Here's how the part is built. I have some questions about the finished solid (model axes, mm). A direction names the side the tool comes from. Coordinates: 2 decimals unless noted, no trailing zeros. Write each loop counter-clockwise with the first axis right and the second up, starting at its lowest first coordinate (ties: lowest second). Pieces come first, ordered by that corner, then holes.
```python
from build123d import *

# Parameters (mm, degrees)
F_5_16_CLEARANCE_HOLE1_D         = 8.4328
CIRPATTERN1_COUNT                = 12
F_1_2_0_5_DIAMETER_HOLE1_D       = 12.7
F_1_1_5_DIAMETER_HOLE1_D         = 38.1
F_1_1_5_DIAMETER_HOLE1_DEPTH     = 19.05
CIRPATTERN2_COUNT                = 6
CIRPATTERN3_COUNT                = 2
F_1_8_0_125_DIAMETER_HOLE1_D     = 3.175
F_1_8_0_125_DIAMETER_HOLE1_DEPTH = 6.35
F_1_8_0_125_DIAMETER_HOLE1_TIP   = 0.953866233


with BuildPart() as part:
    # Sketch1 → Revolve1 (revolve)
    with BuildSketch(Plane.XY, mode=Mode.PRIVATE) as revolve1_sk:
        Polygon((-88.9, 0), (-88.9, 41.275), (-50.8, 41.275), (-31.75, 60.325), (-12.7, 60.325), (-12.7, 53.975), (0, 53.975), (0, 34.925), (-31.75, 34.925), (-31.75, 22.225), (-50.8, 22.225), (-50.8, 3.175), (-52.3875, 3.175), (-52.3875, 5.715), (-55.9435, 5.715), (-55.9435, 3.175), (-57.15, 3.175), (-57.15, 0), align=None)
    revolve(revolve1_sk.sketch.rotate(Axis((0, 0, 0), (0, 1, 0)), 270), axis=Axis((0, 0, 0), (0, 1, 0)))

    # 5/16 Clearance Hole1 (through all)
    with Locations(Plane(origin=(0, 41.275, 0), x_dir=(1, 0, 0), z_dir=(0, 1, 0))):
        with Locations((-73.603547963, -19.722011237)):
            f_5_16_clearance_hole1 = Hole(F_5_16_CLEARANCE_HOLE1_D / 2)

    # CirPattern1: 5/16 Clearance Hole1 ×12 about axis
    cirpattern1_axis = Axis((0, 0, 0), (0, 1, 0))
    for i in range(1, CIRPATTERN1_COUNT):
        add(f_5_16_clearance_hole1.rotate(cirpattern1_axis, i * 360 / CIRPATTERN1_COUNT), mode=Mode.SUBTRACT)

    # 1/2 (0.5) Diameter Hole1 (through all)
    with Locations(Plane(origin=(0, 60.325, 0), x_dir=(1, 0, 0), z_dir=(0, 1, 0))):
        with Locations((0, 0)):
            Hole(F_1_2_0_5_DIAMETER_HOLE1_D / 2)

    # Sketch11 → 1/2 NPT Tapped Hole1 (revolve, cut)
    with BuildSketch(Plane(origin=(41.275, 50.8, 0), x_dir=(-0.707106781186546, 0.707106781186549, 0), z_dir=(0, 0, 1))):
        Polygon((0, 0), (0, 127.968649725), (8.9281, 127.968649725), (8.9281, 13.462), (9.479726792, 13.462), (9.8827971, 0), align=None)
    revolve(axis=Axis((45.765128061, 55.290128061, 0), (-0.707106781186549, -0.707106781186546, 0)), mode=Mode.SUBTRACT)

    # 1 (1.5) Diameter Hole1
    with Locations(Plane(origin=(0, 60.325, 0), x_dir=(1, 0, 0), z_dir=(0, 1, 0))):
        with Locations((-23.8125, -41.244459855)):
            f_1_1_5_diameter_hole1 = Hole(F_1_1_5_DIAMETER_HOLE1_D / 2, depth=F_1_1_5_DIAMETER_HOLE1_DEPTH)

    # Sketch19 → 3/8 NPT Tapped Hole1 (revolve, cut)
    with BuildSketch(Plane(origin=(-23.8125, 41.275, 41.244459855), x_dir=(0, 0, 1), z_dir=(1, 0, 0))):
        Polygon((0, 0), (0, 26.640582582), (7.1374, 22.352), (7.1374, 10.414), (7.653732494, 10.414), (7.9655416, 0), align=None)
    f_3_8_npt_tapped_hole1 = revolve(axis=Axis((-23.8125, 47.625, 41.244459855), (0, -1, 0)), mode=Mode.SUBTRACT)

    # Sketch21 → Tap Drill for 1/4-20 Tap1 (revolve, cut)
    with BuildSketch(Plane(origin=(21.997045256, 60.325, -12.7), x_dir=(0, 0, 1), z_dir=(1, 0, 0))):
        Polygon((0, 0), (0, 17.535816902), (2.5527, 16.002), (2.5527, 0), align=None)
    tap_drill_for_1_4_20_tap1 = revolve(axis=Axis((21.997045256, 66.675, -12.7), (0, -1, 0)), mode=Mode.SUBTRACT)

    # CirPattern2: Tap Drill for 1/4-20 Tap1 ×6 about axis
    cirpattern2_axis = Axis((0, 0, 0), (0, 1, 0))
    for i in range(1, CIRPATTERN2_COUNT):
        add(tap_drill_for_1_4_20_tap1.rotate(cirpattern2_axis, i * 360 / CIRPATTERN2_COUNT), mode=Mode.SUBTRACT)

    # CirPattern3: 1 (1.5) Diameter Hole1, 3/8 NPT Tapped Hole1 ×2 about axis
    cirpattern3_axis = Axis((0, 0, 0), (0, 1, 0))
    add([f_1_1_5_diameter_hole1.rotate(cirpattern3_axis, i * 360 / CIRPATTERN3_COUNT) for i in range(1, CIRPATTERN3_COUNT)], mode=Mode.SUBTRACT)
    add([f_3_8_npt_tapped_hole1.rotate(cirpattern3_axis, i * 360 / CIRPATTERN3_COUNT) for i in range(1, CIRPATTERN3_COUNT)], mode=Mode.SUBTRACT)

    # 1/8 (0.125) Diameter Hole1
    with Locations(Plane(origin=(0, 22.225, 0), x_dir=(-1, 0, 0), z_dir=(0, -1, 0))):
        with Locations((0, 44.45)):
            Hole(F_1_8_0_125_DIAMETER_HOLE1_D / 2, depth=F_1_8_0_125_DIAMETER_HOLE1_DEPTH)
            with Locations((0, 0, -(F_1_8_0_125_DIAMETER_HOLE1_DEPTH + F_1_8_0_125_DIAMETER_HOLE1_TIP / 2))):  # 118° drill point
                Cone(0, F_1_8_0_125_DIAMETER_HOLE1_D / 2, F_1_8_0_125_DIAMETER_HOLE1_TIP, mode=Mode.SUBTRACT)


solid = part.part
```
1) Will these pins go through, and if not, where does the flat tip stop? pin 1 (3 mm diameter, centred on x = -5, y = 9.5, fed in from -Z); pin 2 (13.5 mm diameter, centred on x = 19.72, z = -73.6, fed in from -Y); pin 3 (7.5 mm diameter, centred on x = -53.88, z = -53.88, fed in from +Y); pin 4 (16.5 mm diameter, centred on x = 0, z = 0, fed in from -Y) (3 decimals).
Values follow:
pin 1: stops at z = -88.83
pin 2: stops at y = 0
pin 3: passes through
pin 4: stops at y = 34.925
2) I need wall thicknesses on probe 1 along X at (y, z) = (50, 12.7); probe 2 along X at (y, z) = (12, 52); probe 3 along X at (y, z) = (18, 16.5). Which ranges of each line are inside material? Lowest first, please.
Values follow:
probe 1: x = -40.11 to -24.55, -19.44 to 19.44, 24.55 to 40.11
probe 2: x = -72.11 to -57.65, -50.11 to 50.11, 57.65 to 72.11
probe 3: x = -87.36 to -76.32, -70.88 to -48.05, 48.05 to 70.88, 76.32 to 87.36
3) Imagine slicing it at A-A on x = -71.5. Please give me the cut outline in (y, z) (3 decimals).
Values follow:
outline: (0, -52.83) - (41.275, -52.83) - (41.275, -23.376) - (0, -23.376) - close; (0, -16.068) - (41.275, -16.068) - (41.275, 16.068) - (0, 16.068) - close; (0, 23.376) - (41.275, 23.376) - (41.275, 52.83) - (0, 52.83) - close
4) On a 3-axis mill with a long thin cutter (end or side, diameter ignored), from which of +Z, -Z, +X, -X, +Y, -Y can I reach the whole of each face in a straight line? I mean faces 1 (the face through (-2.513, 1.565, 57.095)), 2 (the face through (14.646, 48.55, -24.545)), 3 (the face through (14, 60.325, 0)). Say none if no direction works.
Values follow:
face 1: -Y
face 2: +Y
face 3: +Z, -Z, +X, -X, +Y
5) We'd pull the mould along Z, two halves only. Please class faces 4 (the face through (58, 0, -1)), 5 (the face through (19.845, 52.436, -11.328)), 6 (the face through (-31.6, 55.2, -19)): pulls with the +Z half, pulls with the -Z half, needs draft (parallel to the pull), parting line crosses it, or undercut.
Values follow:
face 4: needs draft
face 5: undercut
face 6: parting line crosses it
6) Imagine slicing it at B-B on y = 25. Count the separate pieces of the cut face and the enclosed holes in it, then the cut area to 3 significant figures.
Values follow:
separate pieces: 1
enclosed holes: 16
area: 20,700 mm2
